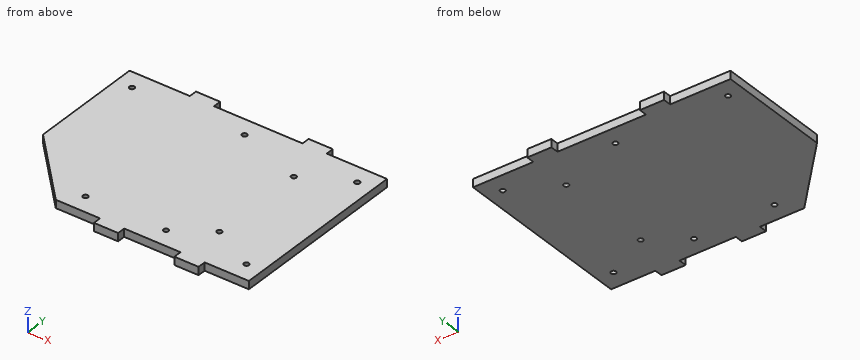
from build123d import *

# Parameters (mm, degrees)
F1_DEPTH = 12.7
F2_D     = 7.9375
F2_DEPTH = 17.4752
F2_TIP   = 2.3846655818


with BuildPart() as f1:
    # F0 (on Top) → F1 (new body)
    with BuildSketch(Plane.XY):
        Polygon((-127, -314.325), (-127, -25.4), (-222.25, -25.4), (-222.25, -12.7), (-260.35, -12.7), (-260.35, -25.4), (-400.05, -25.4), (-400.05, -12.7), (-438.15, -12.7), (-438.15, -25.4), (-533.4, -25.4), (-533.4, -206.375), (-431.8, -314.325), (-361.95, -314.325), (-361.95, -327.025), (-323.85, -327.025), (-323.85, -314.325), (-234.95, -314.325), (-234.95, -327.025), (-196.85, -327.025), (-196.85, -314.325), align=None)
    extrude(amount=F1_DEPTH)

    # F2
    with Locations(Plane(origin=(0, 0, 0), x_dir=(1, 0, 0), z_dir=(0, 0, -1))):
        with Locations((-406.4, 285.75), (-223.8375, 247.65), (-152.4, 285.75), (-279.4, 285.75), (-223.8375, 92.075), (-152.4, 53.975), (-330.2, 53.975), (-508, 53.975)):
            Hole(F2_D / 2, depth=F2_DEPTH)
            with Locations((0, 0, -(F2_DEPTH + F2_TIP / 2))):  # 118° drill point
                Cone(0, F2_D / 2, F2_TIP, mode=Mode.SUBTRACT)


solid = f1.part
The model under review builds one solid part; all positions refer to its coordinate system, in mm. Give positions to 0.01 mm unless a question says otherwise; leave off trailing zeros. Order: outer loops, then holes, each group sorted by start corner. A loop starts at its lowest first (then second) coordinate and runs counter-clockwise, first axis right, second up. Notation, with made-up numbers: M 46.25,-5.75 L 57.25,-5.75 A19 cw 57.25,13.25 Z; hole C -7.5,-17 d7. An arc over 180 degrees is marked long. Use one line per item in the form item = value. Start each with the question number.
Item 1: To check wall thickness, follow line 1 along Y through (x, z) = (-152.4, 10) (3 decimals); line 2 along Y through (x, z) = (-406.4, 7.5) (3 decimals); line 3 along Y through (x, z) = (-294, 12) (3 decimals). State the ranges of each line that lie inside material, in increasing order. Write a range as from..to.
Item 2: Insertion check: pin 1 Ø6.5 at (x, z) = (-350.5, 6) entering from +Y; pin 2 Ø6.5 at (x, y) = (-152.4, -285.75) entering from -Z; pin 3 Ø6.5 at (y, z) = (-323.5, 7.5) entering from -X; pin 4 Ø6.5 at (y, z) = (-21.5, 3.5) entering from +X. Each pin has a flat end and moves straight along its axis. Give the tip position at first contact, or say it passes through.
Item 3: We need section C-C on x = -476. Give the boundary of the cut face in (y, z).
Item 4: We need section A-A on z = 2.25. Give the number of separate pieces and of enclosed holes in the cut face, plus the area to 3 significant figures.
Item 5: We need section B-B on x = -296.5. Give the boundary of the cut face in (y, z) (3 decimals), plus the area to 3 significant figures.
Completed:
q1.line_1 = -314.325..-289.719, -281.781..-57.944, -50.006..-25.4
q1.line_2 = -314.325..-289.719, -281.781..-12.7
q1.line_3 = -314.325..-25.4
q2.pin_1 = -25.4
q2.pin_2 = through
q2.pin_3 = -361.95
q2.pin_4 = -222.25
q3.outline = M -267.36,0 L -25.4,0 L -25.4,12.7 L -267.36,12.7 Z
q4.separate_pieces = 1
q4.enclosed_holes = 8
q4.area = 113,000 mm²
q5.outline = M -314.325,0 L -25.4,0 L -25.4,12.7 L -314.325,12.7 Z
q5.area = 3,670 mm²
